Geometry check sheet. Reference: drawing and pictorial views, mm from the part's lowest x, y, z. Round coordinates to 2 decimals unless told otherwise and drop trailing zeros. Order: outer loops, then holes, each group sorted by start corner. A loop starts at its lowest first (then second) coordinate and runs counter-clockwise, first axis right, second up.
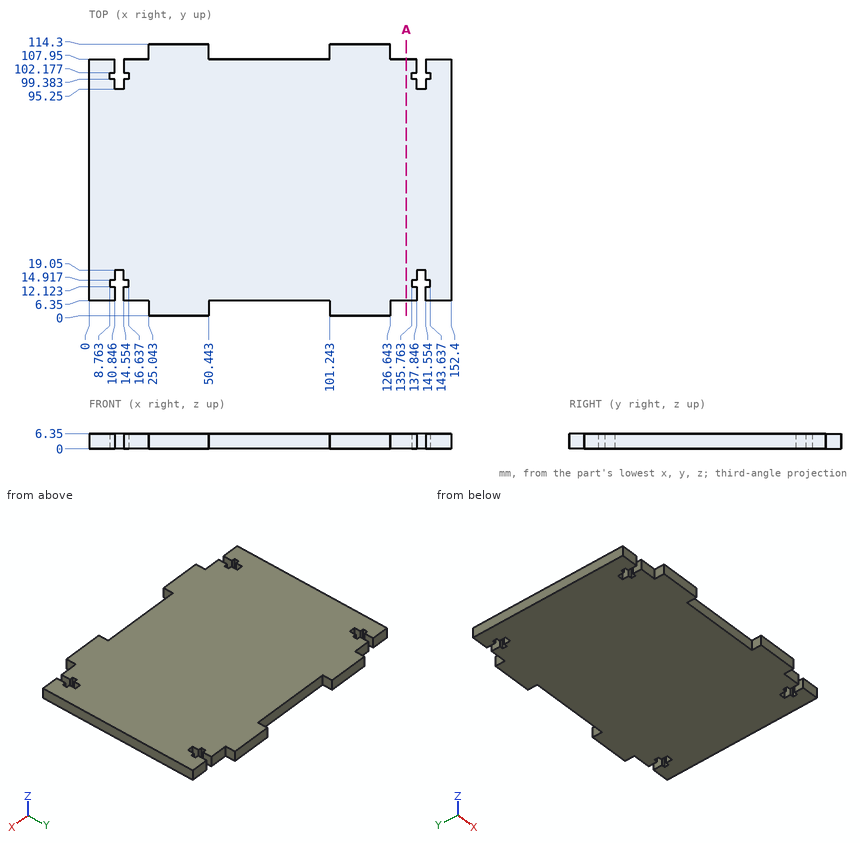
1) Scan lines: probe 1 along X at (y, z) = (16, 2.5) (1 decimal); probe 2 along X at (y, z) = (13.5, 4.5); probe 3 along Y at (x, z) = (69, 1.5). Record each from-to range of solid material in increasing order.
2) Sectioned sample at A-A on x = 133.5. Record the cut outline in (y, z).
3) Go/stop test with flat-tipped pins: pin 1 Ø1.7 at (x, z) = (143, 2) entering from +Y; pin 2 Ø0.6 at (x, z) = (15.5, 3) entering from -Y. Record where each tip stops, or that it passes through.
Returned:
1. probe 1: x = 0 to 10.8, 14.6 to 137.8, 141.6 to 152.4
1. probe 2: x = 0 to 8.76, 16.64 to 135.76, 143.64 to 152.4
1. probe 3: y = 6.35 to 107.95
2. outline: (6.35, 0) - (107.95, 0) - (107.95, 6.35) - (6.35, 6.35) - close
3. pin 1: stops at y = 107.95
3. pin 2: stops at y = 6.35
